Geometry: final body of the model. Coordinates: model frame, mm. A direction names the side the tool comes from. Round coordinates to 2 decimals unless told otherwise and drop trailing zeros. Loops run counter-clockwise (first coordinate to the right, second up) from the corner with the lowest first, then second, coordinate; pieces in that order, holes last. Notation, with made-up numbers: (-21.75, 78.5) - (-13.75, 78.5) arc R17 cw to (-13.75, 93.5) - close; hole circle Ø3 at (10.25, 26.5). An arc over 180 degrees is marked (long way). Answer as CSV lines item,"result".
from build123d import *

# Parameters (mm, degrees)
SKETCH1_R           = 10
SKETCH1_R_2         = 4.3
BOSS_EXTRUDE2_DEPTH = 30
CUT_EXTRUDE1_DEPTH  = 7
BOSS_EXTRUDE3_START = -10
SKETCH3_R           = 15
SKETCH3_R_2         = 10
BOSS_EXTRUDE3_DEPTH = 10
FILLET1_R           = 2.5
FILLET2_R           = 5
SKETCH4_R           = 3
BOSS_EXTRUDE4_DEPTH = 10


with BuildPart() as part:
    # Sketch1 → Boss-Extrude2 (new body)
    with BuildSketch(Plane.XY):
        Circle(SKETCH1_R)
        Circle(SKETCH1_R_2, mode=Mode.SUBTRACT)
    extrude(amount=BOSS_EXTRUDE2_DEPTH)

    # Sketch2 → Cut-Extrude1 (cut)
    with BuildSketch(Plane.XY.offset(30)):
        Polygon((0, 7.505553499), (-6.5, 3.75277675), (-6.5, -3.75277675), (0, -7.505553499), (6.5, -3.75277675), (6.5, 3.75277675), align=None)
    extrude(amount=-CUT_EXTRUDE1_DEPTH, mode=Mode.SUBTRACT)

    # Sketch3 → Boss-Extrude3 (add)
    with BuildSketch(Plane.XY.offset(30).offset(BOSS_EXTRUDE3_START)):
        Circle(SKETCH3_R)
        Circle(SKETCH3_R_2, mode=Mode.SUBTRACT)
    extrude(amount=BOSS_EXTRUDE3_DEPTH)

    # Fillet1
    fillet1_edges = [part.edges().sort_by_distance(p)[0] for p in [
        (-10, 0, 20),
        (-15, 0, 20),
    ]]
    fillet(fillet1_edges, radius=FILLET1_R - 0.0001)  # a hair under: the kernel refuses the full size

    # Fillet2
    fillet2_edges = [part.edges().sort_by_distance(p)[0] for p in [
        (-10, 0, 0),
    ]]
    fillet(fillet2_edges, radius=FILLET2_R)

    # Sketch4 → Boss-Extrude4 (add)
    with BuildSketch(Plane.XY.offset(30)):
        with Locations((11.25277675, 0)):
            Circle(SKETCH4_R)
        with BuildLine():
            ThreePointArc((3, 11.25277675), (2.121320344, 13.374097093), (0, 14.25277675))
            Line((0, 14.25277675), (0, 8.25277675))
            ThreePointArc((0, 8.25277675), (2.121320344, 9.131456406), (3, 11.25277675))
        make_face()
        with BuildLine():
            Line((0, 8.25277675), (0, 14.25277675))
            ThreePointArc((0, 14.25277675), (-3, 11.25277675), (0, 8.25277675))
        make_face()
        with Locations((-11.25277675, 0)):
            Circle(SKETCH4_R)
        with Locations((0, -11.25277675)):
            Circle(SKETCH4_R)
    extrude(amount=BOSS_EXTRUDE4_DEPTH)


solid = part.part
(1) Access query for faces 1 (the face through (-11, 0, 40)), 2 (the face through (3, -6, 30)). Directions: +Z, -Z, +X, -X, +Y, -Y. A direction counts if a zero-diameter tool reaches every point of the face in a straight line with its end or side. Return the directions, or none.
Findings below:
face 1,"+Z, +X, -X, +Y, -Y"
face 2,"+Z"
(2) Section A-A (z = 26). Output: boundary loops of the cut face in (x, y), and give its area (4 significant figures).
Findings below:
outline,"circle Ø30 at (0, 0); hole (-6.5, -3.75) - (0, -7.51) - (6.5, -3.75) - (6.5, 3.75) - (0, 7.51) - (-6.5, 3.75) - close"
area,"560.5 mm2"
(3) Section B-B (z = 18). Output: boundary loops of the cut face in (x, y).
Findings below:
outline,"circle Ø20.1 at (0, 0); hole circle Ø8.6 at (0, 0)"
(4) Pin query (flat end, axial travel): P1, Ø3, axis at y = 2, z = 11, coming from the +X side; P2, Ø6, axis at y = -7, z = 9.5, coming from the +X side; P3, Ø5, axis at y = -11, z = 9, coming from the -X side; P4, Ø5.5, axis at y = 1.5, z = 25, coming from the -X side. Return the tip coordinate at first contact, or that it passes through.
Findings below:
P1,"x = 9.99"
P2,"x = 9.17"
P3,"x = -5.27"
P4,"x = -15"
(5) Draft query along X for faces 3 (the face through (0, 11, 40)), 4 (the face through (-6.5, 0, 27)), 5 (the face through (1.384, -13.914, 34.93)), 6 (the face through (-3.3, -5.6, 26.5)). Return one class per face: pulls with the +X half, pulls with the -X half, needs draft (parallel to the pull), parting line crosses it, or undercut.
Findings below:
face 3,"needs draft"
face 4,"undercut"
face 5,"parting line crosses it"
face 6,"undercut"
(6) Material intervals for line 1 along Y through (x, z) = (0, 8.5); line 2 along Z through (x, y) = (-11.5, -5); line 3 along X through (y, z) = (-11, 33), sorted ascending.
Findings below:
line 1,"-10 to -4.3, 4.3 to 10"
line 2,"20 to 30"
line 3,"-2.99 to 2.99"
